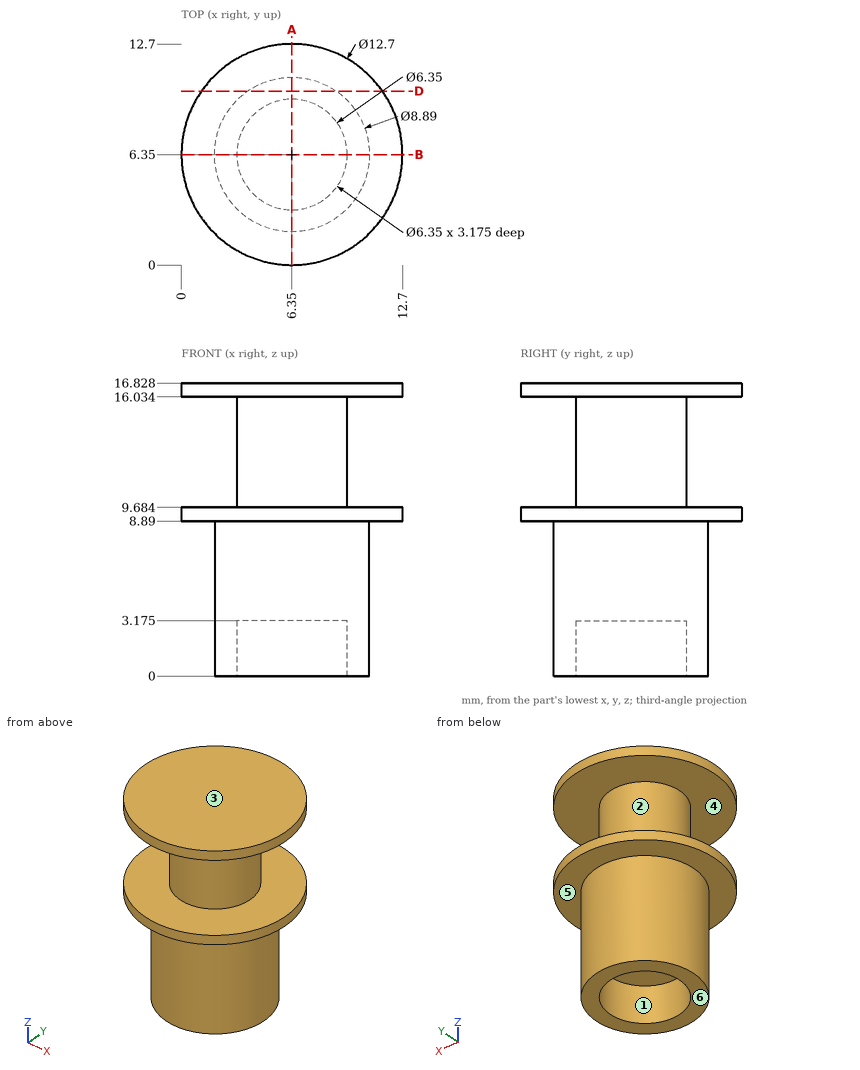
For this review, use the dimensioned drawing (mm, ordinates from the lowest corner) and the shaded views. A direction names the side the tool comes from. Coordinates: 2 decimals unless noted, no trailing zeros. Write each loop counter-clockwise with the first axis right and the second up, starting at its lowest first coordinate (ties: lowest second). Pieces come first, ordered by that corner, then holes. Notation, with made-up numbers: (49, 19) -> (96, 19) arc R14 cw to (96, 38) -> close; hole circle Ø8 at (44, -13). An arc over 180 degrees is marked (long way). Put each result on its own line as item: value.
Q1. Take a section at A-A, the plane x = 6.35. State the section outline as (y, z) points (1 decimal), then the cut area to 3 significant figures.
From the geometry:
outline: (0, 8.9) -> (1.9, 8.9) -> (1.9, 0) -> (3.2, 0) -> (3.2, 3.2) -> (9.5, 3.2) -> (9.5, 0) -> (10.8, 0) -> (10.8, 8.9) -> (12.7, 8.9) -> (12.7, 9.7) -> (9.5, 9.7) -> (9.5, 16) -> (12.7, 16) -> (12.7, 16.8) -> (0, 16.8) -> (0, 16) -> (3.2, 16) -> (3.2, 9.7) -> (0, 9.7) -> close
area: 119 mm2
Q2. The part is to be moulded in two halves that separate along X. For the marked faces 1, 2 and 3, say which applies: +X half, -X half, draft (parallel to the pull), parting line (faces both ways), or undercut.
From the geometry:
face 1: undercut
face 2: parting line
face 3: draft
Q3. Take a section at D-D, the plane y = 10. State the section outline as (x, z) points.
From the geometry:
outline: (1.15, 8.89) -> (3.81, 8.89) -> (3.81, 0) -> (8.89, 0) -> (8.89, 8.89) -> (11.55, 8.89) -> (11.55, 9.68) -> (1.15, 9.68) -> close; (1.15, 16.03) -> (11.55, 16.03) -> (11.55, 16.83) -> (1.15, 16.83) -> close
Q4. Wall thickness on L1, parallel to Z at x = 0.75, y = 6; L2, parallel to Y at x = 6.35, z = 1.45 (1 decimal); L3, parallel to Z at x = 2, y = 6: over which ranges is each line inside the solid? List them lowest first.
From the geometry:
L1: z = 8.89 to 9.68, 16.03 to 16.83
L2: y = 1.9 to 3.2, 9.5 to 10.8
L3: z = 0 to 9.68, 16.03 to 16.83
Q5. Clearance check with flat-ended pins moving along their axes: pin 1 Ø5 at (x, z) = (8.5, 6) entering from +Y (1 decimal); pin 2 Ø2 at (x, z) = (11, 6.5) entering from -Y (1 decimal); pin 3 Ø3 at (y, z) = (9.5, 8) entering from -X (1 decimal). State where each tip first meets the part, or that it passes through.
From the geometry:
pin 1: stops at y = 10.8
pin 2: stops at y = 3.8
pin 3: stops at x = 0.3
Q6. Tool access review of the marked faces 4, 5 and 6: name each direction out of +Z, -Z, +X, -X, +Y, -Y from which nothing blocks a thin tool from reaching the whole face with its end or side.
From the geometry:
face 4: none
face 5: -Z
face 6: -Z, +X, -X, +Y, -Y
